```python
from build123d import *

# Parameters (mm, degrees)
EXTRUDE_2_DEPTH             = 2
M3X0_5_1_D                  = 2.5
M3X0_5_1_DEPTH              = 4
M3X0_5_1_TIP                = 0.751075774
M3X0_5_1_ON_FACE_2_D        = 2.5
M3X0_5_1_ON_FACE_2_DEPTH    = 4
M3X0_5_1_ON_FACE_2_TIP      = 0.751075774
PATTERN_LINEAR_1_COUNT      = 2
PATTERN_LINEAR_1_PITCH      = 98
PATTERN_LINEAR_1_COUNT_DIR2 = 2
PATTERN_LINEAR_1_PITCH_DIR2 = 44
FILLET_4_R                  = 3


with BuildPart() as part:
    # 草圖10 → 填料-伸長2 (new body)
    with BuildSketch(Plane(origin=(0, 0, 0), x_dir=(1, 0, 0), z_dir=(0, 1, 0))):
        with BuildLine():
            Line((56.568542495, 34), (-56.568542495, 34))
            ThreePointArc((-56.568542495, 34), (-61.540159626, 23.849711805), (-64.707032075, 13))
            Line((-64.707032075, 13), (-56.707032075, 13))
            Line((-56.707032075, 13), (-56.707032075, -12.973279994))
            Line((-56.707032075, -12.973279994), (-64.707032075, -13))
            ThreePointArc((-64.707032075, -13), (-61.540159626, -23.849711805), (-56.568542495, -34))
            Line((-56.568542495, -34), (56.568542495, -34))
            ThreePointArc((56.568542495, -34), (61.619473981, -23.644035746), (64.792427449, -12.567471713))
            Line((64.792427449, -12.567471713), (56.707032075, -12.594476939))
            Line((56.707032075, -12.594476939), (56.707032075, 13))
            Line((56.707032075, 13), (64.707032075, 13))
            ThreePointArc((64.707032075, 13), (61.540159626, 23.849711805), (56.568542495, 34))
        make_face()
    extrude(amount=EXTRUDE_2_DEPTH)

    # M3x0.5  螺絲攻的螺孔鑽1
    with Locations(Plane(origin=(30, 2, 30), x_dir=(0, 0, 1), z_dir=(0, 1, 0))):
        with Locations((0, 0), (-60, -60), (0, -60), (-60, 0)):
            Hole(M3X0_5_1_D / 2, depth=M3X0_5_1_DEPTH)
            with Locations((0, 0, -(M3X0_5_1_DEPTH + M3X0_5_1_TIP / 2))):  # 118° drill point
                Cone(0, M3X0_5_1_D / 2, M3X0_5_1_TIP, mode=Mode.SUBTRACT)

    # M3x0.5  螺絲攻的螺孔鑽1 on face 2
    with Locations(Plane(origin=(-30, 0, -30), x_dir=(0, 0, -1), z_dir=(0, -1, 0))):
        with Locations((0, 0)):
            Hole(M3X0_5_1_ON_FACE_2_D / 2, depth=M3X0_5_1_ON_FACE_2_DEPTH)
            with Locations((0, 0, -(M3X0_5_1_ON_FACE_2_DEPTH + M3X0_5_1_ON_FACE_2_TIP / 2))):  # 118° drill point
                Cone(0, M3X0_5_1_ON_FACE_2_D / 2, M3X0_5_1_ON_FACE_2_TIP, mode=Mode.SUBTRACT)

    # 草圖14 → M3x0.5  螺絲攻的螺孔鑽2 (revolve, cut)
    with BuildSketch(Plane(origin=(-49, 2, -22), x_dir=(0, 0, 1), z_dir=(1, 0, 0))):
        Polygon((0, 0), (0, 4.751075774), (1.25, 4), (1.25, 0), align=None)
    m3x0_5_2 = revolve(axis=Axis((-49, 8.35, -22), (0, -1, 0)), mode=Mode.SUBTRACT)

    # 直線複製排列1: M3x0.5 _2 2 × 2
    with Locations(*[(i * PATTERN_LINEAR_1_PITCH, 0, j * PATTERN_LINEAR_1_PITCH_DIR2) for i in range(PATTERN_LINEAR_1_COUNT) for j in range(PATTERN_LINEAR_1_COUNT_DIR2) if (i, j) != (0, 0)]):
        add(m3x0_5_2, mode=Mode.SUBTRACT)

    # 圓角4
    fillet_4_edges = [part.edges().sort_by_distance(p)[0] for p in [
        (-56.707032075, 1, -13),
        (-64.707032075, 1, -13),
        (-56.568542495, 1, -34),
        (56.568542495, 1, -34),
        (64.707032075, 1, -13),
        (56.707032075, 1, -13),
        (56.707032075, 1, 12.594476939),
        (64.792427449, 1, 12.567471713),
        (56.568542495, 1, 34),
        (-56.568542495, 1, 34),
        (-64.707032075, 1, 13),
        (-56.707032075, 1, 12.973279994),
    ]]
    fillet(fillet_4_edges, radius=FILLET_4_R)


solid = part.part
```
For this review, take the finished solid that the model builds, in its own axes (mm). A direction names the side the tool comes from. Round coordinates to 2 decimals unless told otherwise and drop trailing zeros. Write each loop counter-clockwise with the first axis right and the second up, starting at its lowest first coordinate (ties: lowest second). Pieces come first, ordered by that corner, then holes. Notation, with made-up numbers: (74.25, 69.5) -> (124.25, 69.5) arc R22 ccw to (124.25, 77.5) -> close; hole circle Ø8 at (27, 23). An arc over 180 degrees is marked (long way). One line per question, with ' | ' between items. Start each with the question number.
(1) Add section C-C, the plane z = 22. Write out the cut boundary in (x, y), plus the area to 3 significant figures.
(2) Add section A-A, the plane x = 49. Write out the cut boundary in (y, z).
(3) For line 1 along Z through (x, y) = (-49, 1.05); line 2 along X through (y, z) = (1.4, -30); line 3 along X through (y, z) = (0.9, -22), list the stretches that pass through material, from the lowest coordinate up. Write a range as from..to.
(4) Add section D-D, the plane z = -1. Write out the cut boundary in (x, y).
(5) Insertion check: P1, Ø1, axis at x = -60, y = 0.5, coming from the +Z side; P2, Ø0.6, axis at y = 1, z = -3, coming from the +X side. Each pin has a flat end and moves straight along its axis. Give the tip position at first contact, or say it passes through.
(6) Tool access review of faces 1 (the face through (61.2, 0.99, -24.71)), 2 (the face through (57.609, 1.014, -12.145)), 3 (the face through (-57.56, 1.01, 12.08)): name each direction out of +Z, -Z, +X, -X, +Y, -Y from which nothing blocks a thin tool from reaching the whole face with its end or side.
(7) Mouldability with a two-part tool opening along X and no side actions: class faces 4 (the face through (63.333, 1.014, -14.198)), 5 (the face through (-61.2, 0.99, 24.71)), 6 (the face through (47.76, 1.01, -22.16)) as released by +X, released by -X, zero draft, split by the parting line, or undercut.
(8) Add section B-B, the plane y = 0.3. Give the number of separate pieces and of enclosed holes in the cut face, plus the area to 3 significant figures.
Answer list:
1) outline: (-62.23, 0) -> (-50.25, 0) -> (-50.25, 2) -> (-62.23, 2) -> close; (-47.75, 0) -> (47.75, 0) -> (47.75, 2) -> (-47.75, 2) -> close; (50.25, 0) -> (62.23, 0) -> (62.23, 2) -> (50.25, 2) -> close | area: 239 mm²
2) outline: (0, -34) -> (2, -34) -> (2, -23.25) -> (0, -23.25) -> close; (0, -20.75) -> (2, -20.75) -> (2, 20.75) -> (0, 20.75) -> close; (0, 23.25) -> (2, 23.25) -> (2, 34) -> (0, 34) -> close
3) line 1: -34..-23.25, -20.75..20.75, 23.25..34 | line 2: -58.79..-31.25, -28.75..28.75, 31.25..58.79 | line 3: -62.23..-50.25, -47.75..47.75, 50.25..62.23
4) outline: (-56.71, 0) -> (56.71, 0) -> (56.71, 2) -> (-56.71, 2) -> close
5) P1: z = 28.56 | P2: x = 56.71
6) face 1: -Z, +X, +Y, -Y | face 2: +X, +Y, -Y | face 3: -X, +Y, -Y
7) face 4: released by +X | face 5: released by -X | face 6: undercut
8) separate pieces: 1 | enclosed holes: 8 | area: 8,060 mm²
